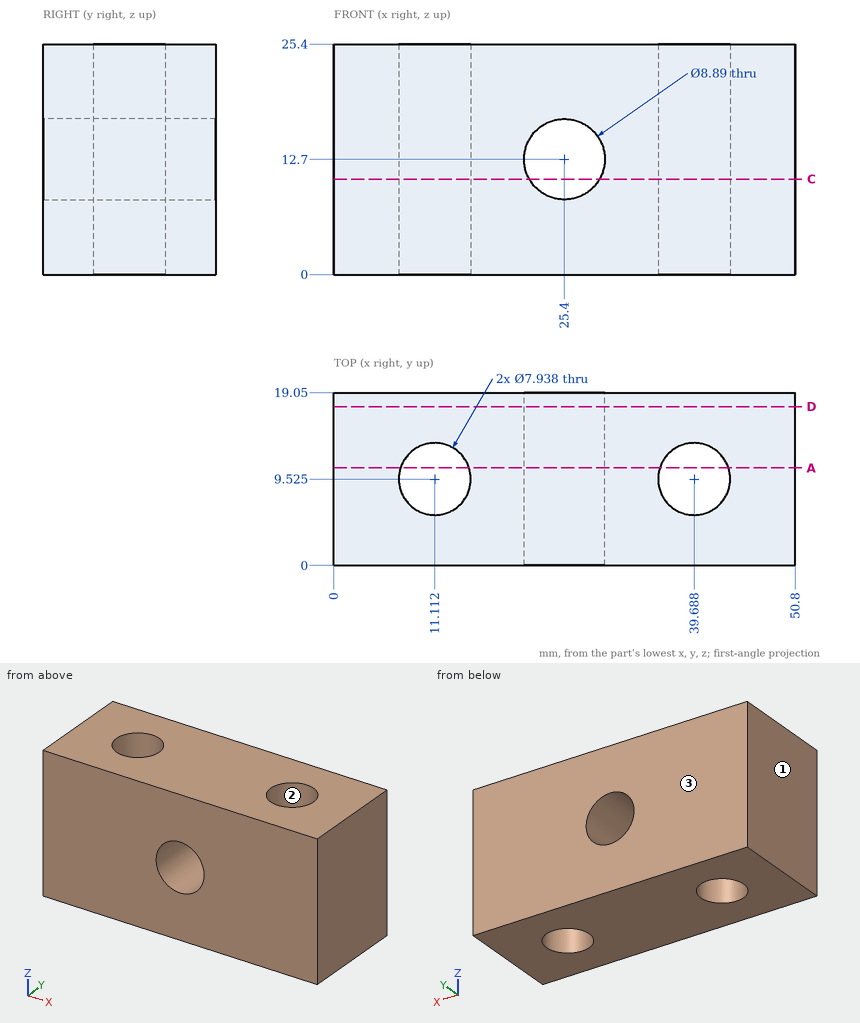
Source: three-view drawing plus pictorial views. Frame: mm from the lowest corner of the part. Give positions to 0.01 mm unless a question says otherwise; leave off trailing zeros. Order: outer loops, then holes, each group sorted by start corner. A loop starts at its lowest first (then second) coordinate and runs counter-clockwise, first axis right, second up. Notation, with made-up numbers: M 3,-29 L 37,-29 A24 ccw 37,-13 Z; hole C 5,26 d10. An arc over 180 degrees is marked long. One line per question, with ' | ' between items. Start each with the question number.
1. Section query D-D (y = 17.5). Return the cut outline in (x, z) (1 decimal), and give its area (3 significant figures).
2. Pull-direction query (Y, two-part tool) for the marked faces 1, 2 and 3; classes: released by +Y, released by -Y, zero draft, split by the parting line, or undercut.
3. Section query A-A (y = 10.75). Return the cut outline in (x, z) (1 decimal).
4. First-contact query: pin 1 Ø1 at (x, y) = (42.5, 9) entering from +Z. Flat tip, straight axial feed; report the tip coordinate or a pass-through.
5. Section query C-C (z = 10.5). Count the separate pieces of the cut face and the enclosed holes in it.
6. Material intervals for probe 1 along Y at (x, z) = (40, 19); probe 2 along X at (y, z) = (8.5, 19); probe 3 along X at (y, z) = (12.75, 6.25) (1 decimal), sorted ascending. Write a range as [from, to].
Here are the results:
1) outline: M 0,0 L 50.8,0 L 50.8,25.4 L 0,25.4 Z; hole C 25.4,12.7 d8.9 | area: 1,230 mm²
2) face 1: zero draft | face 2: undercut | face 3: released by +Y
3) outline: M 0,0 L 7.3,0 L 7.3,25.4 L 0,25.4 Z; M 14.9,0 L 35.9,0 L 35.9,25.4 L 14.9,25.4 Z; M 43.5,0 L 50.8,0 L 50.8,25.4 L 43.5,25.4 Z; hole C 25.4,12.7 d8.9
4) pin 1: through
5) separate pieces: 2 | enclosed holes: 2
6) probe 1: [0, 5.57], [13.48, 19.05] | probe 2: [0, 7.28], [14.95, 35.85], [43.52, 50.8] | probe 3: [0, 8.8], [13.4, 37.4], [42, 50.8]
